```python
from build123d import *

# Parameters (mm, degrees)
F1_DEPTH = 6
F3_DEPTH = 6
F5_DEPTH = 6


with BuildPart() as f1:
    # F0 (on Front) → F1 (new body)
    with BuildSketch(Plane.XZ):
        with BuildLine():
            Line((32, 12.5), (-32, 12.5))
            Line((-32, 12.5), (-32, -12.5))
            Line((-32, -12.5), (32, -12.5))
            Line((32, -12.5), (32, -6.5))
            Line((32, -6.5), (12, -6.5))
            ThreePointArc((12, -6.5), (5.5, 0), (12, 6.5))
            Line((12, 6.5), (32, 6.5))
            Line((32, 6.5), (32, 12.5))
        make_face()
    extrude(amount=F1_DEPTH)

    # F2 (on face) → F3 (join)
    with BuildSketch(Plane(origin=(-32, 0, 0), x_dir=(0, -1, 0), z_dir=(-1, 0, 0))):
        with BuildLine():
            Line((6, -12.5), (6, 12.5))
            Line((6, 12.5), (-12, 12.5))
            ThreePointArc((-12, 12.5), (-3.1611652352, 8.8388347648), (0.5, 0))
            ThreePointArc((0.5, 0), (-3.1611652352, -8.8388347648), (-12, -12.5))
            Line((-12, -12.5), (6, -12.5))
        make_face()
        with BuildLine():
            ThreePointArc((0.5, 0), (-3.1611652352, 8.8388347648), (-12, 12.5))
            Line((-12, 12.5), (-12, 6.5))
            ThreePointArc((-12, 6.5), (-7.4038059223, 4.5961940777), (-5.5, 0))
            ThreePointArc((-5.5, 0), (-7.4038059223, -4.5961940777), (-12, -6.5))
            Line((-12, -6.5), (-12, -12.5))
            ThreePointArc((-12, -12.5), (-3.1611652352, -8.8388347648), (0.5, 0))
        make_face()
        with BuildLine():
            Line((-12, 6.5), (-12, 12.5))
            ThreePointArc((-12, 12.5), (-24.5, 0), (-12, -12.5))
            Line((-12, -12.5), (-12, -6.5))
            ThreePointArc((-12, -6.5), (-18.5, 0), (-12, 6.5))
        make_face()
    extrude(amount=F3_DEPTH)

    # F4 (on face) → F5 (join)
    with BuildSketch(Plane(origin=(0, 0, -12.5), x_dir=(1, 0, 0), z_dir=(0, 0, -1))):
        with BuildLine():
            ThreePointArc((-13, 21.4638169855), (-25.5, 33.9638169855), (-38, 21.4638169855))
            Line((-38, 21.4638169855), (-32, 21.4638169855))
            ThreePointArc((-32, 21.4638169855), (-25.5, 27.9638169855), (-19, 21.4638169855))
            Line((-19, 21.4638169855), (-13, 21.4638169855))
        make_face()
        with BuildLine():
            Line((-32, 21.4638169855), (-38, 21.4638169855))
            ThreePointArc((-38, 21.4638169855), (-25.5, 8.9638169855), (-13, 21.4638169855))
            Line((-13, 21.4638169855), (-19, 21.4638169855))
            ThreePointArc((-19, 21.4638169855), (-25.5, 14.9638169855), (-32, 21.4638169855))
        make_face()
        Polygon((-38, 6), (-38, 0), (-32, 0), (-13, 0), (-13, 6), align=None)
        with BuildLine():
            Line((-38, 21.4638169855), (-38, 6))
            Line((-38, 6), (-13, 6))
            Line((-13, 6), (-13, 21.4638169855))
            ThreePointArc((-13, 21.4638169855), (-25.5, 8.9638169855), (-38, 21.4638169855))
        make_face()
    extrude(amount=-F5_DEPTH)


solid = f1.part
```
CAD build for the part. Positions are in the model's coordinates, mm. A direction names the side the tool comes from. Round coordinates to 2 decimals unless told otherwise and drop trailing zeros. Order: outer loops, then holes, each group sorted by start corner. A loop starts at its lowest first (then second) coordinate and runs counter-clockwise, first axis right, second up. Notation, with made-up numbers: (-20.5, 54.25) - (19.5, 54.25) arc R34 cw to (19.5, 89.25) - close; hole circle Ø1 at (12, 38). An arc over 180 degrees is marked (long way). Answer in a Markdown table with one row per item. Add a question column.
(1) Probe L1, parallel to Y at x = -25.5, z = -8.6; L2, parallel to X at y = 3, z = 1; L3, parallel to Y at x = 7.5, z = 7.25. List the from-to ranges inside material, lowest first. Write a range as [from, to].
(2) 3-axis set-ups, long thin cutter, end or side, ignore diameter. For faces 4 (the face through (22, -3, -6.5)), 5 (the face through (-26, -14, -6.5)), 6 (the face through (-13, -14, -10)), 7 (the face through (-8, 0, 0)): which of +Z, -Z, +X, -X, +Y, -Y reach the whole face in a straight line?
(3) Mould opens along Z. For faces 1 (the face through (-10, -1, 12.5)), 2 (the face through (5.5, -3, -0.1)), 3 (the face through (-25.23, -33.96, -9.54)) say: +Z half, -Z half, draft (parallel to the pull), parting line (faces both ways), or undercut.
(4) Band-saw the part on A-A on x = 14.5. List the corners of the cut face in (y, z).
(5) Drop flat-ended pins along their axis: pin 1 Ø1.8 at (y, z) = (-12, -10) entering from +X; pin 2 Ø6 at (x, z) = (0, 2) entering from -Y; pin 3 Ø1 at (x, z) = (-29, 7.5) entering from +Y. Give the stop position or say it passes through.
(6) Band-saw the part on D-D on z = 5. List the corners of the cut face in (x, y), and give its area (3 significant figures).
(7) Band-saw the part on C-C on y = 17.5. List the corners of the cut face in (x, z), and give its area (3 significant figures).
(8) Band-saw the part on B-B on y = -1. List the corners of the cut face in (x, z).
Data:
| question | item | result |
|---|---|---|
| 1 | L1 | y = [-33.96, -27.96], [-14.96, 0] |
| 1 | L2 | x = [-38, -32] |
| 1 | L3 | y = [-6, 0] |
| 2 | face 4 | +X, +Y, -Y |
| 2 | face 5 | +Z, +X, -X, -Y |
| 2 | face 6 | +Z, -Z, +X, -Y |
| 2 | face 7 | +Z, -Z, +X, +Y |
| 3 | face 1 | +Z half |
| 3 | face 2 | undercut |
| 3 | face 3 | draft |
| 4 | outline | (-6, -12.5) - (0, -12.5) - (0, -6.5) - (-6, -6.5) - close; (-6, 6.5) - (0, 6.5) - (0, 12.5) - (-6, 12.5) - close |
| 5 | pin 1 | stops at x = -13 |
| 5 | pin 2 | stops at y = -6 |
| 5 | pin 3 | stops at y = 0 |
| 6 | outline | (-38, -6) - (7.85, -6) - (7.85, 0) - (-32, 0) - (-32, 7.85) - (-38, 7.85) - close; (-38, 16.15) - (-32, 16.15) - (-32, 23.46) - (-38, 23.46) - close |
| 6 | area | 366 mm^2 |
| 7 | outline | (-38, -11.22) - (-32, -11.22) - (-32, -3.46) - (-38, -3.46) - close; (-38, 3.46) - (-32, 3.46) - (-32, 11.22) - (-38, 11.22) - close |
| 7 | area | 93.1 mm^2 |
| 8 | outline | (-38, -12.5) - (32, -12.5) - (32, -6.5) - (12, -6.5) arc R6.5 cw to (12, 6.5) - (32, 6.5) - (32, 12.5) - (-38, 12.5) - close |
